Autodesk Inventor part; units mm, degrees
ref_plane "YZ Plane" through (0, 0, 0) normal (1, 0, 0) x (0, 1, 0)
ref_plane "XZ Plane" through (0, 0, 0) normal (0, 1, 0) x (-1, 0, 0)
ref_plane "XY Plane" through (0, 0, 0) normal (0, 0, 1) x (1, 0, 0)
sketch "Sketch4" plane through (0, 0, 0) normal (0, 1, 0) x (-1, 0, 0)
  line L0 (0, 0) -> (20, 0)
  line L1 (20, 0) -> (20, -20)
  line L2 (20, -20) -> (0, -20)
  line L3 (0, -20) -> (0, 0)
  dimension "d16" = 20
  dimension "d17" = 20
extrude "Extrusion4" add sketch "Sketch4" along normal blind 38.5
sketch "Sketch5" plane through (-20, 0, 0) normal (0, 0, 1) x (1, 0, 0)
  line L0 (0, 0) -> (0, 38.5)
  line L1 (20, 0) -> (20, 38.5)
  line L2 (0, 10.5) -> (20, 10.5)
  line L3 (20, 10.5) -> (20, 8)
  line L4 (20, 8) -> (0, 8)
  line L5 (0, 8) -> (0, 10.5)
  dimension "d20" = 2.5
  dimension "d21" = 8
extrude "Extrusion5" add sketch "Sketch5" along normal blind 7.5
sketch "Sketch6" plane through (-20, 10.5, 0) normal (0, 1, 0) x (1, 0, 0)
  circle A0 centre (5, -5) radius 2
  circle A1 centre (15, -5) radius 2
  line L0 (0, 0) -> (20, 0)
  line L1 (0, 0) -> (0, -7.5)
  line L2 (20, 0) -> (20, -7.5)
  dimension "d24" = 4
  dimension "d25" = 4
  dimension "d26" = 5
  dimension "d27" = 5
  dimension "d28" = 5
  dimension "d29" = 5
extrude "Extrusion6" cut sketch "Sketch6" against normal through all
mirror "Mirror1" about plane through (0, 0, -20) normal (0, 0, -1)
properties part number "servo"
The model under review builds one solid part; all positions refer to its coordinate system, in mm. A direction names the side the tool comes from. Coordinates: 2 decimals unless noted, no trailing zeros. Write each loop counter-clockwise with the first axis right and the second up, starting at its lowest first coordinate (ties: lowest second). Pieces come first, ordered by that corner, then holes. Notation, with made-up numbers: (1, 39) -> (37, 39) arc R24 cw to (37, 64) -> close; hole circle Ø8 at (23, 29.5). An arc over 180 degrees is marked (long way). Answer in a Markdown table with one row per item.
1. For faces 5 (the flat face through (-10, 8, -44)), 6 (the flat face through (-10, 24, -40)), 7 (the flat face through (-10, 8, 4)), list the 3-axis set-ups (+Z, -Z, +X, -X, +Y, -Y) from which the entire face can be reached by the end or side of a thin tool; tool diameter is ignored.
Answers below:
| item | result |
|---|---|
| face 5 | -Z, +X, -X, -Y |
| face 6 | -Z, +X, -X, +Y |
| face 7 | +Z, +X, -X, -Y |
2. We need section B-B, the plane x = -5. State the section outline as (y, z) points.
Answers below:
| item | result |
|---|---|
| outline | (0, -40) -> (8, -40) -> (8, -43) -> (10.5, -43) -> (10.5, -40) -> (38.5, -40) -> (38.5, 0) -> (10.5, 0) -> (10.5, 3) -> (8, 3) -> (8, 0) -> (0, 0) -> close; (8, -47.5) -> (10.5, -47.5) -> (10.5, -47) -> (8, -47) -> close; (8, 7) -> (10.5, 7) -> (10.5, 7.5) -> (8, 7.5) -> close |
3. Wall thickness on probe 1 along Z at (x, y) = (-5, 9.6); probe 2 along Z at (x, y) = (-4.25, 10); probe 3 along Z at (x, y) = (-3, 20): over which ranges is each line inside the solid? List them lowest first. Write a range as [from, to].
Answers below:
| item | result |
|---|---|
| probe 1 | z = [-47.5, -47], [-43, 3], [7, 7.5] |
| probe 2 | z = [-47.5, -46.85], [-43.15, 3.15], [6.85, 7.5] |
| probe 3 | z = [-40, 0] |
4. We need section D-D, the plane y = 34. State the section outline as (x, z) points, and give its area (3 significant figures).
Answers below:
| item | result |
|---|---|
| outline | (-20, -40) -> (0, -40) -> (0, 0) -> (-20, 0) -> close |
| area | 800 mm^2 |
5. We need section C-C, the plane x = -11. State the section outline as (y, z) points, and give its area (3 significant figures).
Answers below:
| item | result |
|---|---|
| outline | (0, -40) -> (8, -40) -> (8, -47.5) -> (10.5, -47.5) -> (10.5, -40) -> (38.5, -40) -> (38.5, 0) -> (10.5, 0) -> (10.5, 7.5) -> (8, 7.5) -> (8, 0) -> (0, 0) -> close |
| area | 1,580 mm^2 |
6. Clearance check with flat-ended pins moving along their axes: pin 1 Ø6 at (x, y) = (-14, 27) entering from -Z; pin 2 Ø2.5 at (x, z) = (-15, -45) entering from +Y; pin 3 Ø1 at (x, y) = (-7.5, 19) entering from +Z; pin 4 Ø2 at (x, z) = (-6.5, 3.5) entering from +Y. State where each tip first meets the part, or that it passes through.
Answers below:
| item | result |
|---|---|
| pin 1 | stops at z = -40 |
| pin 2 | passes through |
| pin 3 | stops at z = 0 |
| pin 4 | stops at y = 10.5 |
7. We need section A-A, the plane z = 5. State the section outline as (x, y) points.
Answers below:
| item | result |
|---|---|
| outline | (-20, 8) -> (-17, 8) -> (-17, 10.5) -> (-20, 10.5) -> close; (-13, 8) -> (-7, 8) -> (-7, 10.5) -> (-13, 10.5) -> close; (-3, 8) -> (0, 8) -> (0, 10.5) -> (-3, 10.5) -> close |
8. Draft analysis for pull direction X (two halves, no side actions). For faces 1 (the cylindrical face through (-6.6, 9.3, 6.2)), 2 (the flat face through (-20, 19, -20)), 3 (the flat face through (-10, 0, -20)), 4 (the cylindrical face through (-5, 9, -43)), state which applies: +X half, -X half, draft (parallel to the pull), parting line (faces both ways), or undercut.
Answers below:
| item | result |
|---|---|
| face 1 | undercut |
| face 2 | -X half |
| face 3 | draft |
| face 4 | undercut |
